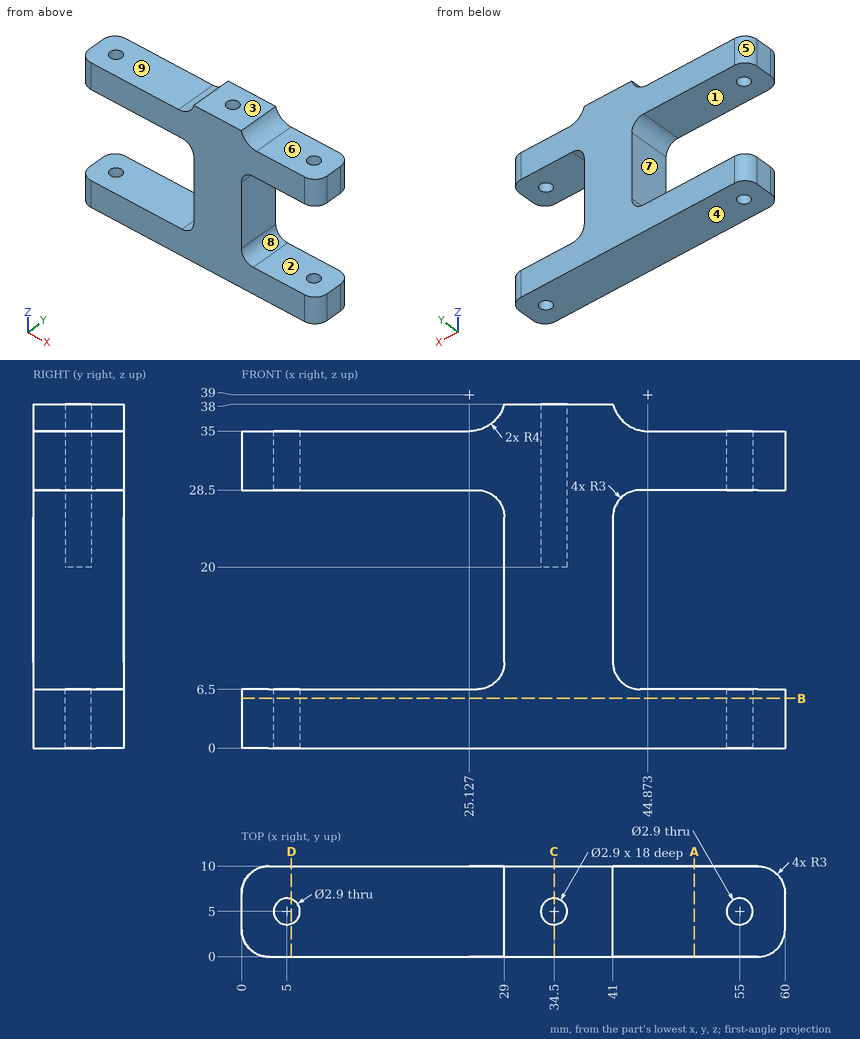
Geometry check sheet. Reference: drawing and pictorial views, mm from the part's lowest x, y, z. A direction names the side the tool comes from. Round coordinates to 2 decimals unless told otherwise and drop trailing zeros. Write each loop counter-clockwise with the first axis right and the second up, starting at its lowest first coordinate (ties: lowest second). Pieces come first, ordered by that corner, then holes.
1. Draft check along Z on the marked faces 1, 2, 3 and 4. Enter one of: +Z half, -Z half, draft (parallel to the pull), parting line (faces both ways), or undercut.
2. Section check C-C on x = 34.5. Enter the section's corners in (y, z).
3. Gauge pin test, flat ends, axial feed: P1, Ø3, axis at x = 13, y = 4, coming from the +Z side; P2, Ø3, axis at y = 3.5, z = 10.5, coming from the +X side; P3, Ø1.5, axis at y = 4, z = 18.5, coming from the -X side. Record the tip position at first contact, or that the pin passes through.
4. Section check B-B on z = 5.5. Enter the section's corners in (x, y), plus the area to 3 significant figures.
5. Access from +Z, -Z, +X, -X, +Y, -Y to the whole of each face (thin tool, end or side, straight path). Record for the marked faces 5, 6, 7, 8 and 9.
6. Section check D-D on x = 5.5. Enter the section's corners in (y, z), plus the area to 3 significant figures.
7. Scan lines: L1, parallel to Z at x = 50, y = 9.25; L2, parallel to Y at x = 5, z = 31; L3, parallel to X at y = 5.25, z = 33. Record each from-to range of solid material in increasing order.
8. Section check A-A on x = 50. Enter the section's corners in (y, z), plus the area to 3 significant figures.
Answer:
1. face 1: undercut
1. face 2: undercut
1. face 3: +Z half
1. face 4: -Z half
2. outline: (0, 0) - (10, 0) - (10, 38) - (6.45, 38) - (6.45, 20) - (3.55, 20) - (3.55, 38) - (0, 38) - close
3. P1: stops at z = 35
3. P2: stops at x = 41.04
3. P3: stops at x = 29
4. outline: (0, 3) arc R3 ccw to (3, 0) - (57, 0) arc R3 ccw to (60, 3) - (60, 7) arc R3 ccw to (57, 10) - (3, 10) arc R3 ccw to (0, 7) - close; hole circle Ø2.9 at (5, 5); hole circle Ø2.9 at (55, 5)
4. area: 579 mm2
5. face 5: +Z, -Z, -X, +Y
5. face 6: +Z, +X, +Y, -Y
5. face 7: -X, +Y, -Y
5. face 8: +X, +Y, -Y
5. face 9: +Z, -X, +Y, -Y
6. outline: (0, 0) - (3.64, 0) - (3.64, 6.5) - (0, 6.5) - close; (0, 28.5) - (3.64, 28.5) - (3.64, 35) - (0, 35) - close; (6.36, 0) - (10, 0) - (10, 6.5) - (6.36, 6.5) - close; (6.36, 28.5) - (10, 28.5) - (10, 35) - (6.36, 35) - close
6. area: 94.6 mm2
7. L1: z = 0 to 6.5, 28.5 to 35
7. L2: y = 0 to 3.55, 6.45 to 10
7. L3: x = 0 to 3.57, 6.43 to 33.07, 35.93 to 53.57, 56.43 to 60
8. outline: (0, 0) - (10, 0) - (10, 6.5) - (0, 6.5) - close; (0, 28.5) - (10, 28.5) - (10, 35) - (0, 35) - close
8. area: 130 mm2
